Read the model definition and answer for the solid it produces. Units are mm, in the model's axes. Give positions to 0.01 mm unless a question says otherwise; leave off trailing zeros. Loops run counter-clockwise (first coordinate to the right, second up) from the corner with the lowest first, then second, coordinate; pieces in that order, holes last. Notation, with made-up numbers: (34.25, -12) - (92.25, -12) arc R8 ccw to (92.25, -3) - close; hole circle Ø5 at (-5, 1.25). An arc over 180 degrees is marked (long way). Write item = value, one per line.
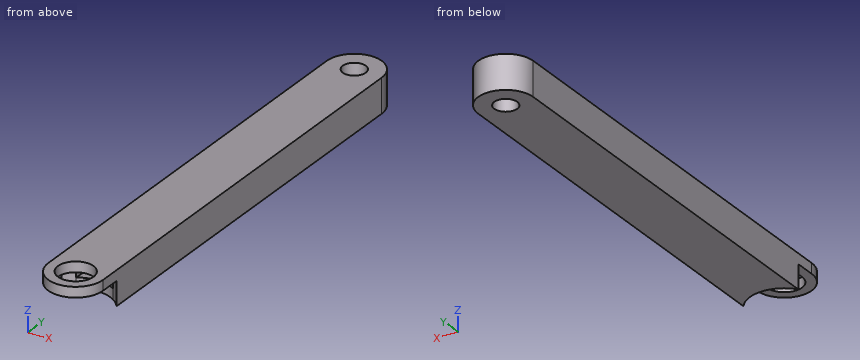
```python
from build123d import *

# Parameters (mm, degrees)
SKETCH1_R           = 1.700000029
BOSS_EXTRUDE1_DEPTH = 5.08
CUT_EXTRUDE1_START  = -2.54
CUT_EXTRUDE1_DEPTH  = 1.016
SKETCH3_R           = 2.6289
CUT_EXTRUDE2_DEPTH  = 2.032
CUT_EXTRUDE3_REACH  = 7.08
SKETCH2_3_R         = 1.700000029


with BuildPart() as part:
    # Sketch1 → Boss-Extrude1 (new body)
    with BuildSketch(Plane(origin=(-856.488519717, 635.703940982, 371.824950285), x_dir=(1, 0, 0), z_dir=(0, 0, 1))):
        with BuildLine():
            Line((4.064, 31.75), (4.064, -31.75))
            ThreePointArc((4.064, -31.75), (0, -35.814), (-4.064, -31.75))
            Line((-4.064, -31.75), (-4.064, 31.75))
            ThreePointArc((-4.064, 31.75), (0, 35.814), (4.064, 31.75))
        make_face()
        with Locations((0, -31.75)):
            Circle(SKETCH1_R, mode=Mode.SUBTRACT)
        with Locations((0, 31.75)):
            Circle(SKETCH1_R, mode=Mode.SUBTRACT)
    extrude(amount=BOSS_EXTRUDE1_DEPTH)

    # Sketch2 → Cut-Extrude1 (cut, symmetric)
    with BuildSketch(Plane(origin=(0, 0, 371.824950285), x_dir=(-1, 0, 0), z_dir=(0, 0, -1)).offset(CUT_EXTRUDE1_START)):
        with BuildLine():
            Line((859.219019717, 608.237720826), (858.581157709, 620.429720826))
            ThreePointArc((858.581157709, 620.429720826), (856.488519717, 622.415738028), (854.395881724, 620.429720826))
            Line((854.395881724, 620.429720826), (853.758019717, 608.237720826))
            ThreePointArc((853.758019717, 608.237720826), (856.488519717, 598.873940982), (859.219019717, 608.237720826))
        make_face()
    extrude(amount=CUT_EXTRUDE1_DEPTH, both=True, mode=Mode.SUBTRACT)

    # Sketch3 → Cut-Extrude2 (cut)
    with BuildSketch(Plane(origin=(0, 0, 375.380950285), x_dir=(-1, 0, 0), z_dir=(0, 0, -1))):
        with Locations((856.488519717, 603.953940982)):
            Circle(SKETCH3_R)
    extrude(amount=-CUT_EXTRUDE2_DEPTH, mode=Mode.SUBTRACT)

    # Sketch2_3 → Cut-Extrude3 (cut, up to next)
    with BuildSketch(Plane(origin=(0, 0, 371.824950285), x_dir=(-1, 0, 0), z_dir=(0, 0, -1)), mode=Mode.PRIVATE) as cut_extrude3_sk1:
        with BuildLine():
            ThreePointArc((860.552519717, 607.001940982), (859.941503284, 607.679971642), (859.219019717, 608.237720826))
            ThreePointArc((859.219019717, 608.237720826), (856.488519717, 609.033940982), (853.758019717, 608.237720826))
            ThreePointArc((853.758019717, 608.237720826), (853.035536149, 607.679971642), (852.424519717, 607.001940982))
            Line((852.424519717, 607.001940982), (852.424519717, 603.953940982))
            ThreePointArc((852.424519717, 603.953940982), (856.488519717, 599.889940982), (860.552519717, 603.953940982))
            Line((860.552519717, 603.953940982), (860.552519717, 607.001940982))
        make_face()
        with Locations((856.488519717, 603.953940982)):
            Circle(SKETCH2_3_R, mode=Mode.SUBTRACT)
    cut_extrude3_tool1 = extrude(cut_extrude3_sk1.sketch, amount=-CUT_EXTRUDE3_REACH, mode=Mode.PRIVATE) & part.part
    add(cut_extrude3_tool1.solids().sort_by_distance((-859.858344, 607.590237, 371.82495))[0], mode=Mode.SUBTRACT)


solid = part.part
```
1) A cutting plane is placed at C-C on x = -856.25. Determine the outline of the cut face in (y, z), then the cut area to 3 significant figures.
Output:
outline = (599.9, 375.38) - (601.34, 375.38) - (601.34, 376.9) - (599.9, 376.9) - close; (606.57, 375.38) - (622.4, 375.38) - (622.4, 373.35) - (609.03, 373.35) - (609.03, 371.82) - (665.77, 371.82) - (665.77, 376.9) - (606.57, 376.9) - close; (669.14, 371.82) - (671.51, 371.82) - (671.51, 376.9) - (669.14, 376.9) - close
area = 279 mm²
2) A cutting plane is placed at D-D on z = 376. Determine the outline of the cut face in (x, y), then the cut area to 3 significant figures.
Output:
outline = (-860.55, 603.95) arc R4.06 ccw to (-852.42, 603.95) - (-852.42, 667.45) arc R4.06 ccw to (-860.55, 667.45) - close; hole circle Ø5.26 at (-856.49, 603.95); hole circle Ø3.4 at (-856.49, 667.45)
area = 537 mm²
3) A cutting plane is placed at B-B on y = 610. Determine the outline of the cut face in (x, z).
Output:
outline = (-860.55, 371.82) - (-852.42, 371.82) - (-852.42, 376.9) - (-860.55, 376.9) - close; hole (-859.13, 373.35) - (-853.85, 373.35) - (-853.85, 375.38) - (-859.13, 375.38) - close
4) A cutting plane is placed at A-A on z = 372.5. Determine the outline of the cut face in (x, y).
Output:
outline = (-860.55, 607) arc R5.08 cw to (-852.42, 607) - (-852.42, 667.45) arc R4.06 ccw to (-860.55, 667.45) - close; hole circle Ø3.4 at (-856.49, 667.45)
5) Find the intervals of material crossed by probe 1 along Y at (x, z) = (-855, 375.55); probe 2 along Z at (x, y) = (-856.25, 617); probe 3 along Y at (x, z) = (-857.75, 375.7), in increasing order.
Output:
probe_1 = 600.17 to 601.79, 606.12 to 666.63, 668.28 to 671.24
probe_2 = 371.82 to 373.35, 375.38 to 376.9
probe_3 = 600.09 to 601.65, 606.26 to 666.31, 668.59 to 671.32
